The model under review builds one solid part; all positions refer to its coordinate system, in mm. Face numbers are marked on the shaded views. A direction names the side the tool comes from. Round coordinates to 2 decimals unless told otherwise and drop trailing zeros. Loops run counter-clockwise (first coordinate to the right, second up) from the corner with the lowest first, then second, coordinate; pieces in that order, holes last. Notation, with made-up numbers: (2.25, 37) -> (31.25, 37) arc R7 cw to (31.25, 41) -> close; hole circle Ø2 at (-18.5, -39.5). An arc over 180 degrees is marked (long way). Write each question's results on one line, items separated by ' | '. Start each with the question number.
Item 1: We need section B-B (x = 16). Give the boundary of the cut face in (y, z), and give its area (3 significant figures).
Item 2: For L1, parallel to Z at x = 17.5, y = -16.75; L2, parallel to X at y = -10.5, z = 10.5; L3, parallel to Z at x = 64.5, y = -1.5, list the stretches that pass through material, from the lowest coordinate up. Write a range as from..to.
Item 3: We need section A-A (y = -5.25). Give the boundary of the cut face in (x, z), and give its area (4 significant figures).
Item 4: Clearance check with flat-ended pins moving along their axes: pin 1 Ø9 at (x, y) = (4.5, -8) entering from -Z; pin 2 Ø10 at (x, z) = (22.5, 27.5) entering from +Y; pin 3 Ø5.5 at (y, z) = (-7.5, 6) entering from -X. State where each tip first meets the part, or that it passes through.
Item 5: Tool access review of the marked faces 1 and 2: name each direction out of +Z, -Z, +X, -X, +Y, -Y from which nothing blocks a thin tool from reaching the whole face with its end or side.
Item 6: We need section C-C (z = 9). Give the boundary of the cut face in (x, y).
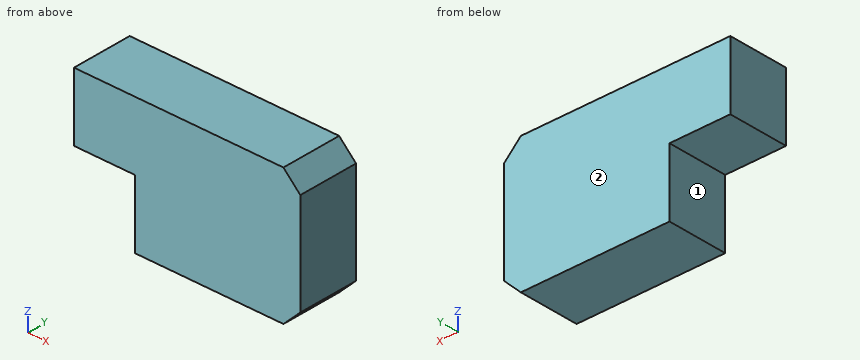
from build123d import *

# Parameters (mm, degrees)
F1_DEPTH = 18
F2_SIZE  = 5


with BuildPart() as f1:
    # F0 (on Front) → F1 (new body)
    with BuildSketch(Plane.XZ):
        Polygon((18, 20), (18, 0), (67, 0), (67, 40), (0, 40), (0, 20), align=None)
    extrude(amount=F1_DEPTH)

    # F2
    f2_edges = [f1.edges().sort_by_distance(p)[0] for p in [
        (67, -9, 40),
        (67, -9, 0),
    ]]
    chamfer(f2_edges, length=F2_SIZE)


solid = f1.part
Here are the results:
1) outline: (-18, 20) -> (0, 20) -> (0, 40) -> (-18, 40) -> close | area: 360 mm2
2) L1: z = 20..40 | L2: x = 18..67 | L3: z = 2.5..37.5
3) outline: (0, 20) -> (18, 20) -> (18, 0) -> (62, 0) -> (67, 5) -> (67, 35) -> (62, 40) -> (0, 40) -> close | area: 2,295 mm2
4) pin 1: stops at z = 20 | pin 2: stops at y = 0 | pin 3: stops at x = 18
5) face 1: -Z, -X, +Y, -Y | face 2: +Z, -Z, +X, -X, +Y
6) outline: (18, -18) -> (67, -18) -> (67, 0) -> (18, 0) -> close
